Part print with two shaded views. Sizes in mm from the minimum x, y, z corner. A direction names the side the tool comes from. Give positions to 0.01 mm unless a question says otherwise; leave off trailing zeros. Order: outer loops, then holes, each group sorted by start corner. A loop starts at its lowest first (then second) coordinate and runs counter-clockwise, first axis right, second up. Notation, with made-up numbers: M 33,17.5 L 48,17.5 A34 ccw 48,49.5 Z; hole C 36,72 d5. An arc over 180 degrees is marked long. Answer as CSV lines item,"result".
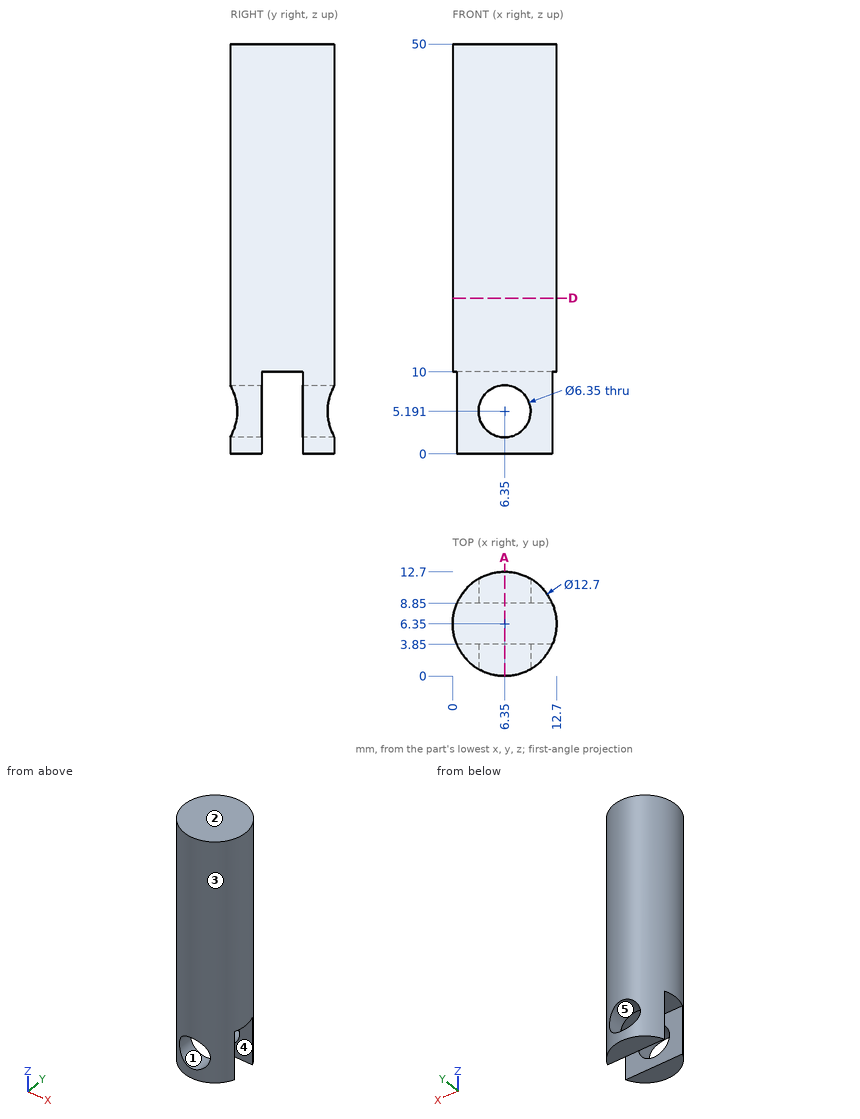
Item 1: Band-saw the part on A-A (x = 6.35). Give the cut face in (y, z), and give its area (3 significant figures).
Geometry says:
outline,"M 0,0 L 3.85,0 L 3.85,2.02 L 0,2.02 Z; M 0,8.37 L 3.85,8.37 L 3.85,10 L 8.85,10 L 8.85,8.37 L 12.7,8.37 L 12.7,50 L 0,50 Z; M 8.85,0 L 12.7,0 L 12.7,2.02 L 8.85,2.02 Z"
area,"536 mm2"
Item 2: Band-saw the part on D-D (z = 19). Give the cut face in (x, y), and give its area (3 significant figures).
Geometry says:
outline,"C 6.35,6.35 d12.7"
area,"127 mm2"
Item 3: 3-axis set-ups, long thin cutter, end or side, ignore diameter. For the marked faces 4 and 5: which of +Z, -Z, +X, -X, +Y, -Y reach the whole face in a straight line?
Geometry says:
face 4,"-Z, +X, -X"
face 5,"+Y, -Y"
Item 4: Pull direction X, two halves, no side cores. Call the marked faces 1, 2 and 3: released by +X, released by -X, zero draft, split by the parting line, or undercut.
Geometry says:
face 1,"undercut"
face 2,"zero draft"
face 3,"split by the parting line"
Item 5: Drop flat-ended pins along their axis: pin 1 (1 mm diameter, centred on y = 7, z = 35.5, fed in from +X); pin 2 (5 mm diameter, centred on x = 8, z = 5.5, fed in from +Y); pin 3 (1.5 mm diameter, centred on x = 9.5, y = 7.5, fed in from -Z); pin 4 (4 mm diameter, centred on x = 6.35, z = 5.19, fed in from -Y). Give the stop position or say it passes through.
Geometry says:
pin 1,"stops at x = 12.7"
pin 2,"stops at y = 12.52"
pin 3,"stops at z = 10"
pin 4,"passes through"
Item 6: Probe line 1 along X through (y, z) = (6, 14); line 2 along Y through (x, z) = (6.5, 45); line 3 along Z through (x, y) = (4.25, 4.5). List the from-to ranges inside material, lowest first. Write a range as from..to.
Geometry says:
line 1,"x = 0.01..12.69"
line 2,"y = 0..12.7"
line 3,"z = 10..50"
